Model file for the job. Use its own axes, mm. Face numbers are marked on the shaded views. Round coordinates to 2 decimals unless told otherwise and drop trailing zeros. Loops run counter-clockwise (first coordinate to the right, second up) from the corner with the lowest first, then second, coordinate; pieces in that order, holes last. Notation, with made-up numbers: (52.25, 27.5) - (77.25, 27.5) arc R14 cw to (77.25, 44.5) - close; hole circle Ø5 at (47.5, 23.5). An arc over 180 degrees is marked (long way). Answer as a JSON object with one key per item and string values.
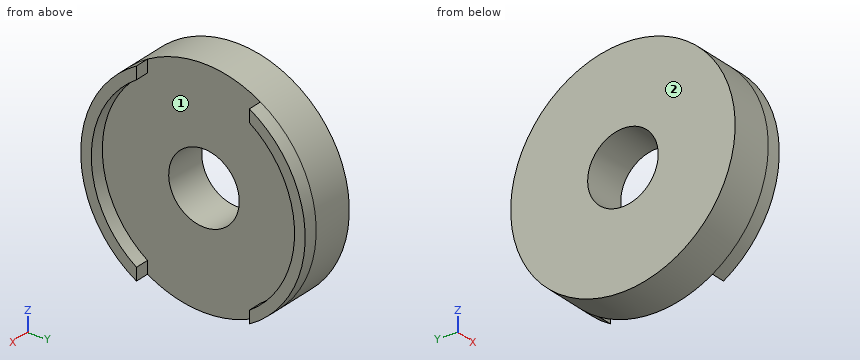
from build123d import *

# Parameters (mm, degrees)
SKETCH1_R           = 15.9
SKETCH1_R_2         = 5
BOSS_EXTRUDE1_DEPTH = 6
BOSS_EXTRUDE2_DEPTH = 2


with BuildPart() as part:
    # Sketch1 → Boss-Extrude1 (new body)
    with BuildSketch(Plane(origin=(0, 0, 0), x_dir=(0, 0, -1), z_dir=(1, 0, 0))):
        Circle(SKETCH1_R)
        Circle(SKETCH1_R_2, mode=Mode.SUBTRACT)
    extrude(amount=BOSS_EXTRUDE1_DEPTH)

    # Sketch2 → Boss-Extrude2 (add)
    with BuildSketch(Plane(origin=(6, 0, 0), x_dir=(0, 0, -1), z_dir=(1, 0, 0))):
        with BuildLine():
            Line((11.973303638, -8), (13.740815114, -8))
            ThreePointArc((13.740815114, -8), (0, -15.9), (-13.740815114, -8))
            Line((-13.740815114, -8), (-11.973303638, -8))
            ThreePointArc((-11.973303638, -8), (0, -14.4), (11.973303638, -8))
        make_face()
        with BuildLine():
            Line((-13.740815114, 8), (-11.973303638, 8))
            ThreePointArc((-11.973303638, 8), (0, 14.4), (11.973303638, 8))
            Line((11.973303638, 8), (13.740815114, 8))
            ThreePointArc((13.740815114, 8), (0, 15.9), (-13.740815114, 8))
        make_face()
    extrude(amount=BOSS_EXTRUDE2_DEPTH)


solid = part.part
1) Slice it at A-A on z = 0. List the corners of the cut face in (x, y), then the cut area to 3 significant figures.
Values follow:
{"outline": "(0, -15.9) - (8, -15.9) - (8, -14.4) - (6, -14.4) - (6, -5) - (0, -5) - close; (0, 5) - (6, 5) - (6, 14.4) - (8, 14.4) - (8, 15.9) - (0, 15.9) - close", "area": "137 mm²"}
2) Drop flat-ended pins along their axis: P1, Ø1.5, axis at x = 5, y = -9, coming from the +Z side; P2, Ø8, axis at y = -1, z = -9.5, coming from the +X side; P3, Ø1.4, axis at x = 7.5, z = 13, coming from the -Y side; P4, Ø6, axis at y = 0, z = 0, coming from the -X side. Give the stop position or say it passes through.
Values follow:
{"P1": "z = 13.59", "P2": "x = 6", "P3": "y = -10.08", "P4": "through"}
3) Slice it at D-D on x = 3.5. List the corners of the cut face in (y, z), then the cut area to 3 significant figures.
Values follow:
{"outline": "circle Ø31.8 at (0, 0); hole circle Ø10 at (0, 0)", "area": "716 mm²"}
4) Slice it at B-B on y = 0. List the corners of the cut face in (x, z).
Values follow:
{"outline": "(0, -15.9) - (6, -15.9) - (6, -5) - (0, -5) - close; (0, 5) - (6, 5) - (6, 15.9) - (0, 15.9) - close"}
5) Probe probe 1 along Y at (x, z) = (3.3, 0); probe 2 along X at (y, z) = (-2, -14); probe 3 along Y at (x, z) = (6.75, -12). List the from-to ranges inside material, lowest first.
Values follow:
{"probe 1": "-15.9 to -5, 5 to 15.9", "probe 2": "0 to 6", "probe 3": "-10.43 to -8, 8 to 10.43"}
6) Two-plate mould, pull along Y, no slides. Class the marked faces 1 and 2: pulls with the +Y half, pulls with the -Y half, needs draft (parallel to the pull), parting line crosses it, or undercut.
Values follow:
{"face 1": "undercut", "face 2": "needs draft"}
7) Slice it at C-C on x = 7.5. List the corners of the cut face in (y, z).
Values follow:
{"outline": "(-8, -13.74) - (-8, -11.97) arc R14.4 cw to (-8, 11.97) - (-8, 13.74) arc R15.9 ccw to start; (8, -13.74) arc R15.9 ccw to (8, 13.74) - (8, 11.97) arc R14.4 cw to (8, -11.97) - close"}
